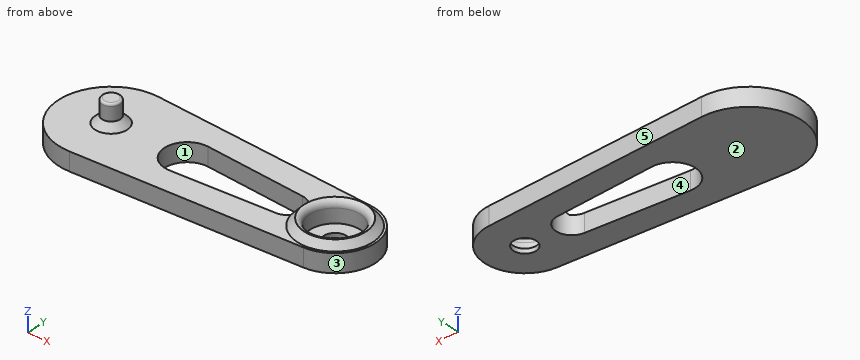
```python
from build123d import *

# Parameters (mm, degrees)
SKETCH5_R           = 4
BOSS_EXTRUDE1_DEPTH = 10
SKETCH13_R          = 5.0000000000000036
BOSS_EXTRUDE5_DEPTH = 8
CHAMFER1_SIZE       = 3
FILLET1_R           = 1
SKETCH14_R          = 13.499999999999998
BOSS_EXTRUDE6_DEPTH = 3.1
CUT_EXTRUDE1_START  = -6
SKETCH15_R          = 11.050000000000002
CUT_EXTRUDE1_DEPTH  = 20
FILLET2_R           = 3
CHAMFER2_SIZE       = 3


with BuildPart() as part:
    # Sketch5 → Boss-Extrude1 (new body)
    with BuildSketch(Plane(origin=(0, 0, 0), x_dir=(0, 1, 0), z_dir=(0, 0, 1))):
        with Locations(Location((0, 0, 0), (0, 0, 270))):
            Circle(SKETCH5_R)
    extrude(amount=BOSS_EXTRUDE1_DEPTH)

    # Sketch13 → Boss-Extrude5 (add)
    with BuildSketch(Plane(origin=(0, 0, 0), x_dir=(0, 1, 0), z_dir=(0, 0, 1))):
        with BuildLine():
            Line((-17.473511202674743, -100.9625), (-22.96518615208682, -1.2650000000000037))
            ThreePointArc((-22.96518615208682, -1.2650000000000037), (1.41e-15, 23.000000000000004), (22.96518615208682, -1.2649999999999981))
            Line((22.96518615208682, -1.2649999999999981), (17.47351120267477, -100.9625))
            ThreePointArc((17.47351120267477, -100.9625), (1.332e-14, -117.5), (-17.473511202674743, -100.9625))
        make_face()
        with Locations(Location((1.225e-14, -100, 0), (0, 0, 270))):
            Circle(SKETCH13_R, mode=Mode.SUBTRACT)
        with BuildLine():
            Line((-9.977753031397176, -34.66666666666667), (-6.984427121978019, -79.46666666666665))
            ThreePointArc((-6.984427121978019, -79.46666666666665), (8.55e-15, -86), (6.9844271219780385, -79.46666666666665))
            Line((6.9844271219780385, -79.46666666666665), (9.977753031397182, -34.66666666666667))
            ThreePointArc((9.977753031397182, -34.66666666666667), (4.78e-15, -24), (-9.977753031397176, -34.66666666666667))
        make_face(mode=Mode.SUBTRACT)
    extrude(amount=-BOSS_EXTRUDE5_DEPTH)

    # Chamfer1
    chamfer1_edges = [part.edges().sort_by_distance(p)[0] for p in [
        (-4, 1.22e-15, 0),
    ]]
    chamfer(chamfer1_edges, length=CHAMFER1_SIZE)

    # Fillet1
    fillet1_edges = [part.edges().sort_by_distance(p)[0] for p in [
        (-4, 1.22e-15, 10),
    ]]
    fillet(fillet1_edges, radius=FILLET1_R)

    # Sketch14 → Boss-Extrude6 (add)
    with BuildSketch(Plane(origin=(0, 0, 0), x_dir=(0, 1, 0), z_dir=(0, 0, 1))):
        with Locations(Location((1.225e-14, -100, 0), (0, 0, 90))):
            Circle(SKETCH14_R)
    extrude(amount=BOSS_EXTRUDE6_DEPTH)

    # Sketch15 → Cut-Extrude1 (cut)
    with BuildSketch(Plane(origin=(0, 0, 0), x_dir=(0, 1, 0), z_dir=(0, 0, 1)).offset(CUT_EXTRUDE1_START)):
        with Locations(Location((1.225e-14, -100, 0), (0, 0, 270))):
            Circle(SKETCH15_R)
    extrude(amount=CUT_EXTRUDE1_DEPTH, mode=Mode.SUBTRACT)

    # Fillet2
    # the kernel refuses this fillet: 3 mm, written as the material it takes off along each edge
    with BuildSketch(Plane(origin=(100, 1.225e-14, 3.0999999999999996), x_dir=(1, -1.8e-16, 0), z_dir=(1.8e-16, 1, 0))) as fillet2_piece_1:
        with BuildLine():
            CenterArc((14.049999999999997, 2.949152420612873), FILLET2_R, 180, 79.43602241094561)
            Line((11.049999999999997, 2.949152420612873), (10.989999999999995, 2.949152420612873))
            Line((10.989999999999995, 2.949152420612873), (10.989999999999995, 0))
            Line((10.989999999999995, 0), (11.049999999999997, -0.06000000000000005))
            ThreePointArc((11.049999999999997, -0.06000000000000005), (12.275000000000105, -0.0600000000000005), (13.489000000000217, -0.05898304841112623))
            Line((13.489000000000217, -0.05898304841112623), (13.500000000000213, 1.10889e-12))
        make_face()
    revolve(axis=Axis((100, 1.225e-14, 3.0999999999999996), (0, 0, -1)), mode=Mode.SUBTRACT)

    # Chamfer2
    # the kernel refuses this chamfer: 3 mm, written as the material it adds along each edge
    with BuildSketch(Plane(origin=(100, 1.225e-14, 0), x_dir=(-1, 6e-17, 0), z_dir=(6e-17, 1, 0))) as chamfer2_piece_1_section:
        Polygon((13.5 + CHAMFER2_SIZE, 0), (13.5, CHAMFER2_SIZE), (13.5, 0), align=None)
    chamfer2_piece_1 = revolve(axis=Axis((100, 1.225e-14, 0), (0, 0, 1)), mode=Mode.PRIVATE)
    chamfer2_piece_1 = chamfer2_piece_1 - Plane(origin=(78.99999999999999, 9.77e-15, 1.4464911380903063), x_dir=(0.0666666666666669, -0.9977753031397177, 0), z_dir=(0, 0, 1)) * Cylinder(7.000000000000007, 66, mode=Mode.PRIVATE)
    add(chamfer2_piece_1)


solid = part.part
```
Verification items for the finished model (mm, model axes). Face numbers are marked on the shaded views. A direction names the side the tool comes from. Round coordinates to 2 decimals unless told otherwise and drop trailing zeros. Order: outer loops, then holes, each group sorted by start corner. A loop starts at its lowest first (then second) coordinate and runs counter-clockwise, first axis right, second up. Notation, with made-up numbers: (-23, -6) - (-17, -6) arc R30 ccw to (-17, 22) - close; hole circle Ø1 at (-10, -1.75). An arc over 180 degrees is marked (long way). Use CSV: the item, a comma, the result in double quotes. Start each with the question number.
1) Section check B-B, the plane x = 46. Record the cut outline in (y, z), plus the area to 3 significant figures.
2) Section check D-D, the plane x = 0. Record the cut outline in (y, z).
3) Mould release check, pull along Y, two halves, no side actions. Record for the marked faces 3, 4 and 5: +Y half, -Y half, draft (parallel to the pull), parting line (faces both ways), or undercut.
4) Access from +Z, -Z, +X, -X, +Y, -Y to the whole of each face (thin tool, end or side, straight path). Record for the marked faces 1 and 2.
5) Thickness scan on L1, parallel to X at y = -4.5, z = -4.25; L2, parallel to Z at x = 108.5, y = 1; L3, parallel to Z at x = 53, y = 17. Record the ranges inside material, lowest first.
6) Section check A-A, the plane z = -3. State how many separate pieces and enclosed holes the cut face has, plus the area to 3 significant figures.
7) Go/stop test with flat-tipped pins: P1, Ø9, axis at x = 100, y = 0, coming from the -Z side; P2, Ø17.5, axis at x = 96.5, y = 3, coming from the +Z side; P3, Ø10, axis at x = 102, z = 6, coming from the -Y side; P4, Ø10, axis at x = 86, z = -4, coming from the -Y side. Record where each tip stops, or that it passes through.
Answers:
1,outline,"(-20.5, -8) - (-9.22, -8) - (-9.22, 0) - (-20.5, 0) - close; (9.22, -8) - (20.5, -8) - (20.5, 0) - (9.22, 0) - close"
1,area,"180 mm²"
2,outline,"(-23, -8) - (23, -8) - (23, 0) - (7, 0) - (4, 3) - (4, 9) arc R1 ccw to (3, 10) - (-3, 10) arc R1 ccw to (-4, 9) - (-4, 3) - (-7, 0) - (-23, 0) - close"
3,face 3,"parting line"
3,face 4,"undercut"
3,face 5,"+Y half"
4,face 1,"+Z, -Z"
4,face 2,"-Z, +X, -X, +Y, -Y"
5,L1,"x = -22.56 to 25.07, 84.36 to 89.91, 110.09 to 116.91"
5,L2,"z = -8 to -6"
5,L3,"z = -8 to 0"
6,separate pieces,"1"
6,enclosed holes,"2"
6,area,"3,980 mm²"
7,P1,"passes through"
7,P2,"stops at z = 3.07"
7,P3,"stops at y = -15.4"
7,P4,"stops at y = -18.57"
